```python
from build123d import *

# Parameters (mm, degrees)
SKETCH1_W           = 8.4
SKETCH1_H           = 28.4
BOSS_EXTRUDE1_DEPTH = 46.4
FILLET1_R           = 3.5
FILLET2_R           = 1.25


with BuildPart() as part:
    # Sketch1 → Boss-Extrude1 (new body)
    with BuildSketch(Plane(origin=(0, 0, 0), x_dir=(1, 0, 0), z_dir=(0, 1, 0))):
        Rectangle(SKETCH1_W, SKETCH1_H)
    extrude(amount=BOSS_EXTRUDE1_DEPTH)

    # Fillet1
    fillet1_edges = [part.edges().sort_by_distance(p)[0] for p in [
        (4.2, 23.2, 14.2),
        (-4.2, 23.2, 14.2),
        (-4.2, 23.2, -14.2),
        (4.2, 23.2, -14.2),
    ]]
    fillet(fillet1_edges, radius=FILLET1_R)

    # Fillet2
    fillet2_edges = [part.edges().sort_by_distance(p)[0] for p in [
        (-4.2, 0, 0),
        (-4.2, 46.4, 0),
        (4.2, 0, 0),
        (0, 0, 14.2),
        (0, 0, -14.2),
        (-3.174873734, 0, 13.174873734),
        (3.174873734, 0, 13.174873734),
        (3.174873734, 0, -13.174873734),
        (-3.174873734, 0, -13.174873734),
        (0, 46.4, -14.2),
        (4.2, 46.4, 0),
        (0, 46.4, 14.2),
        (-3.174873734, 46.4, 13.174873734),
        (3.174873734, 46.4, 13.174873734),
        (3.174873734, 46.4, -13.174873734),
        (-3.174873734, 46.4, -13.174873734),
    ]]
    fillet(fillet2_edges, radius=FILLET2_R)


solid = part.part
```
Geometry: final body of the model. Coordinates: model frame, mm. Round coordinates to 2 decimals unless told otherwise and drop trailing zeros. Write each loop counter-clockwise with the first axis right and the second up, starting at its lowest first coordinate (ties: lowest second). Pieces come first, ordered by that corner, then holes. Notation, with made-up numbers: (-19, 89.5) -> (2, 89.5) arc R25 ccw to (2, 119.5) -> close; hole circle Ø3 at (-20, 13.5). An arc over 180 degrees is marked (long way). Return JSON: item names as keys, results as strings.
Q1. Ray query, line 1 (Y direction, x = -3, z = -5.75); line 2 (Z direction, x = -1.5, y = 26.5); line 3 (Z direction, x = 3.25, y = 10.5). Return the intervals inside material, ascending.
From the geometry:
{"line 1": "0 to 46.4", "line 2": "-14.11 to 14.11", "line 3": "-13.1 to 13.1"}
Q2. Section A-A on y = 41. Return the cut outline in (x, z), and give its area (3 significant figures).
From the geometry:
{"outline": "(-4.2, -10.7) arc R3.5 ccw to (-0.7, -14.2) -> (0.7, -14.2) arc R3.5 ccw to (4.2, -10.7) -> (4.2, 10.7) arc R3.5 ccw to (0.7, 14.2) -> (-0.7, 14.2) arc R3.5 ccw to (-4.2, 10.7) -> close", "area": "228 mm2"}
Q3. First-contact query: pin 1 Ø1 at (x, y) = (3, 11.5) entering from -Z. Flat tip, straight axial feed; report the tip coordinate or a pass-through.
From the geometry:
{"pin 1": "z = -13.7"}
